Can you work these out from the model? Positions are in its coordinate system, mm. A direction names the side the tool comes from. Coordinates: 2 decimals unless noted, no trailing zeros. Write each loop counter-clockwise with the first axis right and the second up, starting at its lowest first coordinate (ties: lowest second). Pieces come first, ordered by that corner, then holes. Notation, with made-up numbers: M 5.5,20 L 9.5,20 A22 cw 9.5,26 Z; hole C 11.25,79.25 d7. An arc over 180 degrees is marked long. Answer as a JSON object with one key per item and string values. Group by question number.
from build123d import *

# Parameters (mm, degrees)
F0_R     = 1.75
F0_W     = 12
F0_H     = 10
F1_DEPTH = 2
F2_R     = 1.75
F3_DEPTH = 1
F4_R     = 2
F5_DEPTH = 34
F6_W     = 8.5
F6_H     = 2
F7_DEPTH = 5


with BuildPart() as f1:
    # F0 (on Top) → F1 (new body)
    with BuildSketch(Plane.XY):
        with BuildLine():
            ThreePointArc((-17, -13), (-15.828427, -15.828427), (-13, -17))
            Line((-13, -17), (13, -17))
            ThreePointArc((13, -17), (15.828427, -15.828427), (17, -13))
            Line((17, -13), (17, 13))
            ThreePointArc((17, 13), (15.828427, 15.828427), (13, 17))
            Line((13, 17), (-13, 17))
            ThreePointArc((-13, 17), (-15.828427, 15.828427), (-17, 13))
            Line((-17, 13), (-17, -13))
        make_face()
        with Locations((-13, -13)):
            Circle(F0_R, mode=Mode.SUBTRACT)
        with Locations((-7, -7)):
            Circle(F0_R, mode=Mode.SUBTRACT)
        with Locations((13, -13)):
            Circle(F0_R, mode=Mode.SUBTRACT)
        with Locations((7, -7)):
            Circle(F0_R, mode=Mode.SUBTRACT)
        with Locations((-7, 7)):
            Circle(F0_R, mode=Mode.SUBTRACT)
        with Locations((-13, 13)):
            Circle(F0_R, mode=Mode.SUBTRACT)
        Rectangle(F0_W, F0_H, mode=Mode.SUBTRACT)
        with Locations((7, 7)):
            Circle(F0_R, mode=Mode.SUBTRACT)
        with Locations((13, 13)):
            Circle(F0_R, mode=Mode.SUBTRACT)
    extrude(amount=F1_DEPTH)

    # F2 (on face) → F3 (join)
    with BuildSketch(Plane.XY.offset(2)):
        with BuildLine():
            ThreePointArc((-17, -13), (-15.828427, -15.828427), (-13, -17))
            Line((-13, -17), (13, -17))
            ThreePointArc((13, -17), (15.828427, -15.828427), (17, -13))
            Line((17, -13), (17, 13))
            ThreePointArc((17, 13), (15.828427, 15.828427), (13, 17))
            Line((13, 17), (-13, 17))
            ThreePointArc((-13, 17), (-15.828427, 15.828427), (-17, 13))
            Line((-17, 13), (-17, -13))
        make_face()
        with Locations((-13, -13)):
            Circle(F2_R, mode=Mode.SUBTRACT)
        with Locations((-7, -7)):
            Circle(F2_R, mode=Mode.SUBTRACT)
        with Locations((13, -13)):
            Circle(F2_R, mode=Mode.SUBTRACT)
        with Locations((7, -7)):
            Circle(F2_R, mode=Mode.SUBTRACT)
        with Locations((-7, 7)):
            Circle(F2_R, mode=Mode.SUBTRACT)
        with Locations((-13, 13)):
            Circle(F2_R, mode=Mode.SUBTRACT)
        with Locations((7, 7)):
            Circle(F2_R, mode=Mode.SUBTRACT)
        with Locations((13, 13)):
            Circle(F2_R, mode=Mode.SUBTRACT)
    extrude(amount=F3_DEPTH)


with BuildPart() as f5:
    # F4 (on face) → F5 (new body)
    with BuildSketch(Plane.XZ.offset(17)):
        with Locations((0, 3)):
            Circle(F4_R)
    extrude(amount=-F5_DEPTH)


with BuildPart() as f7:
    # F6 (on face) → F7 (new body)
    with BuildSketch(Plane.XY.offset(3)):
        Rectangle(F6_W, F6_H)
    extrude(amount=-F7_DEPTH)


with BuildPart() as f1_1:
    add(f1.part)

    # F8: cut F5, F7
    add(f5.part, mode=Mode.SUBTRACT)
    add(f7.part, mode=Mode.SUBTRACT)


solid = f1_1.part
Q1. If we section it at A-A on y = -4.5: List the corners of the cut face in (x, z) for me.
Q2. If we section it at C-C on y = 7: List the corners of the cut face in (x, z) for me, and give its area (3 significant figures).
Q3. We'd pull the mould along Y, two halves only. Please class faces 1 (the flat face through (17, 0, 1)), 2 (the cylindrical face through (-15.797, 15.859, 1.479)), 3 (the cylindrical face through (-6.19, 5.45, 1.48)), 4 (the cylindrical face through (-13.228, -11.265, 1.479)): pulls with the +Y half, pulls with the -Y half, needs draft (parallel to the pull), parting line crosses it, or undercut.
Q4. If we section it at D-D on z = 1.45: Give the number of separate pieces and of enclosed holes in the cut face, and give its area (3 significant figures).
Q5. Will this pin go through, and if not, where does the flat tip stop? pin 1 (1.3 mm diameter, centred on x = 3, y = 1.5, fed in from -Z).
Q6. If we section it at B-B on x = -7: List the corners of the cut face in (y, z) for me, and give its area (3 significant figures).
Q7. On a 3-axis mill with a long thin cutter (end or side, diameter ignored), from which of +Z, -Z, +X, -X, +Y, -Y can I reach the whole of each face in a straight line? I mean faces 5 (the flat face through (-17, 0, 1)), 6 (the flat face through (6, 0, 1)), 7 (the flat face through (3, -1, 2.5)). Say none if no direction works.
Q8. Please list where these lines run through material, in increasing order: L1, parallel to Y at x = -13, z = 1.3; L2, parallel to Y at x = 7, z = 2.15; L3, parallel to Y at x = -1, z = 0.7.
Reply:
{
 "1": {"outline": "M -17,0 L -6,0 L -6,2 L -1.73,2 A2 cw -2,3 L -17,3 Z; M 1.73,2 L 6,2 L 6,0 L 17,0 L 17,3 L 2,3 A2 cw Z"},
 "2": {"outline": "M -17,0 L -8.75,0 L -8.75,3 L -17,3 Z; M -5.25,0 L 5.25,0 L 5.25,3 L 2,3 A2 cw -2,3 L -5.25,3 Z; M 8.75,0 L 17,0 L 17,3 L 8.75,3 Z", "area": "74.7 mm^2"},
 "3": {"face 1": "needs draft", "face 2": "pulls with the +Y half", "face 3": "undercut", "face 4": "undercut"},
 "4": {"separate pieces": "2", "enclosed holes": "8", "area": "885 mm^2"},
 "5": {"pin 1": "z = 2"},
 "6": {"outline": "M -17,0 L -8.75,0 L -8.75,3 L -17,3 Z; M -5.25,0 L 5.25,0 L 5.25,3 L -5.25,3 Z; M 8.75,0 L 17,0 L 17,3 L 8.75,3 Z", "area": "81.0 mm^2"},
 "7": {"face 5": "+Z, -Z, -X, +Y, -Y", "face 6": "-Z", "face 7": "+Z, -Z"},
 "8": {"L1": "-17 to -14.75, -11.25 to 11.25, 14.75 to 17", "L2": "-17 to -8.75, -5.25 to 5.25, 8.75 to 17", "L3": "-17 to -5, 5 to 17"}
}
